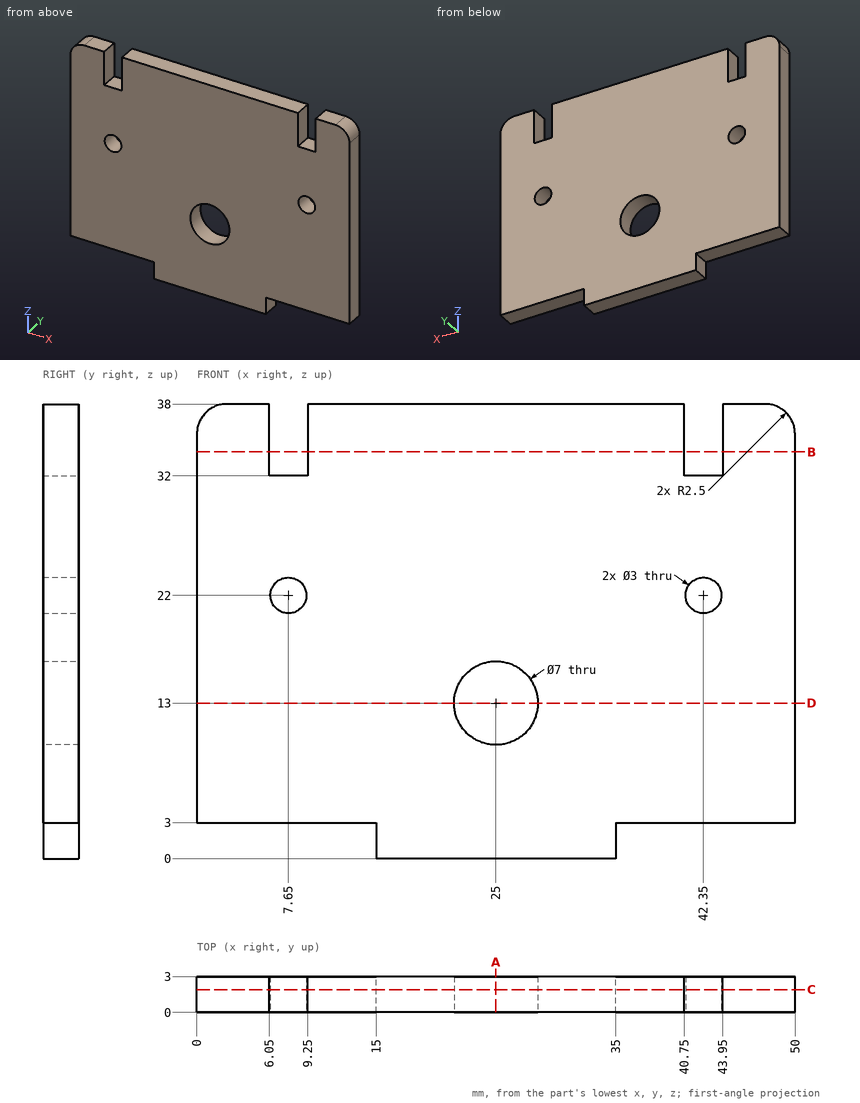
Can you work these out from the drawing? Everything is in mm from the part's minimum corner. Coordinates: 2 decimals unless noted, no trailing zeros. Loops run counter-clockwise (first coordinate to the right, second up) from the corner with the lowest first, then second, coordinate; pieces in that order, holes last. Notation, with made-up numbers: M -28,-31 L -13,-31 A34 ccw -13,1 Z; hole C 51,59.25 d10. An arc over 180 degrees is marked long. One line per item, written item: value.
1. Imagine slicing it at D-D (z = 13). List the corners of the cut face in (x, y) for me, and give its area (3 significant figures).
Geometry says:
outline: M 0,0 L 21.5,0 L 21.5,3 L 0,3 Z; M 28.5,0 L 50,0 L 50,3 L 28.5,3 Z
area: 129 mm2
2. Please list where these lines run through material, in increasing order: probe 1 along X at (y, z) = (2, 35); probe 2 along X at (y, z) = (1.55, 22); probe 3 along Z at (x, y) = (42.35, 1.2).
Geometry says:
probe 1: x = 0 to 6.05, 9.25 to 40.75, 43.95 to 50
probe 2: x = 0 to 6.15, 9.15 to 40.85, 43.85 to 50
probe 3: z = 3 to 20.5, 23.5 to 32
3. Imagine slicing it at A-A (x = 25). List the corners of the cut face in (y, z) for me.
Geometry says:
outline: M 0,0 L 3,0 L 3,9.5 L 0,9.5 Z; M 0,16.5 L 3,16.5 L 3,38 L 0,38 Z
4. Imagine slicing it at B-B (z = 34). List the corners of the cut face in (x, y) for me.
Geometry says:
outline: M 0,0 L 6.05,0 L 6.05,3 L 0,3 Z; M 9.25,0 L 40.75,0 L 40.75,3 L 9.25,3 Z; M 43.95,0 L 50,0 L 50,3 L 43.95,3 Z
5. Imagine slicing it at C-C (y = 1.9). List the corners of the cut face in (x, z) for me, and give its area (3 significant figures).
Geometry says:
outline: M 0,3 L 15,3 L 15,0 L 35,0 L 35,3 L 50,3 L 50,35.5 A2.5 ccw 47.5,38 L 43.95,38 L 43.95,32 L 40.75,32 L 40.75,38 L 9.25,38 L 9.25,32 L 6.05,32 L 6.05,38 L 2.5,38 A2.5 ccw 0,35.5 Z; hole C 7.65,22 d3; hole C 25,13 d7; hole C 42.35,22 d3
area: 1,720 mm2
6. Will these pins go through, and if not, where does the flat tip stop? pin 1 Ø0.9 at (y, z) = (1, 1) entering from -X; pin 2 Ø1.5 at (x, y) = (10, 1.5) entering from -Z.
Geometry says:
pin 1: stops at x = 15
pin 2: stops at z = 3
